Can you work these out from the model? Positions are in its coordinate system, mm. Face numbers are marked on the shaded views. A direction names the side the tool comes from. Round coordinates to 2 decimals unless told otherwise and drop trailing zeros. Loops run counter-clockwise (first coordinate to the right, second up) from the corner with the lowest first, then second, coordinate; pieces in that order, holes last.
from build123d import *

# Parameters (mm, degrees)
SKETCH1_W           = 440
SKETCH1_H           = 327.889328918
BOSS_EXTRUDE1_DEPTH = 120
SKETCH8_W           = 413.828334862
SKETCH8_H           = 293.441910175
CUT_EXTRUDE1_DEPTH  = 110
SKETCH9_R           = 6
SKETCH9_R_2         = 6.017467881
CUT_EXTRUDE4_DEPTH  = 110
SKETCH10_R          = 6
SKETCH10_R_2        = 6.017467881
CUT_EXTRUDE5_DEPTH  = 110


with BuildPart() as part:
    # Sketch1 → Boss-Extrude1 (new body)
    with BuildSketch(Plane(origin=(0, 0, 0), x_dir=(1, 0, 0), z_dir=(0, 1, 0))):
        with Locations((-220, 163.944664459)):
            Rectangle(SKETCH1_W, SKETCH1_H)
    extrude(amount=BOSS_EXTRUDE1_DEPTH)

    # Sketch8 → Cut-Extrude1 (cut)
    with BuildSketch(Plane(origin=(0, 120, 0), x_dir=(1, 0, 0), z_dir=(0, 1, 0))):
        with Locations((-219.994628395, 162.587971533)):
            Rectangle(SKETCH8_W, SKETCH8_H)
    extrude(amount=-CUT_EXTRUDE1_DEPTH, mode=Mode.SUBTRACT)

    # Sketch9 → Cut-Extrude4 (cut)
    with BuildSketch(Plane(origin=(-426.908795826, 0, 0), x_dir=(0, 0, -1), z_dir=(1, 0, 0))):
        with Locations((278, 80)):
            Circle(SKETCH9_R)
        with Locations((278, 26.719560601)):
            Circle(SKETCH9_R)
        with Locations((50, 80)):
            Circle(SKETCH9_R)
        with Locations((50, 26.719560601)):
            Circle(SKETCH9_R_2)
    extrude(amount=-CUT_EXTRUDE4_DEPTH, mode=Mode.SUBTRACT)

    # Sketch10 → Cut-Extrude5 (cut)
    with BuildSketch(Plane(origin=(0, 0, 0), x_dir=(0, 0, -1), z_dir=(1, 0, 0))):
        with Locations((50, 80)):
            Circle(SKETCH10_R)
        with Locations((50, 26.719560601)):
            Circle(SKETCH10_R_2)
        with Locations((278, 26.719560601)):
            Circle(SKETCH10_R)
        with Locations((278, 80)):
            Circle(SKETCH10_R)
    extrude(amount=-CUT_EXTRUDE5_DEPTH, mode=Mode.SUBTRACT)


solid = part.part
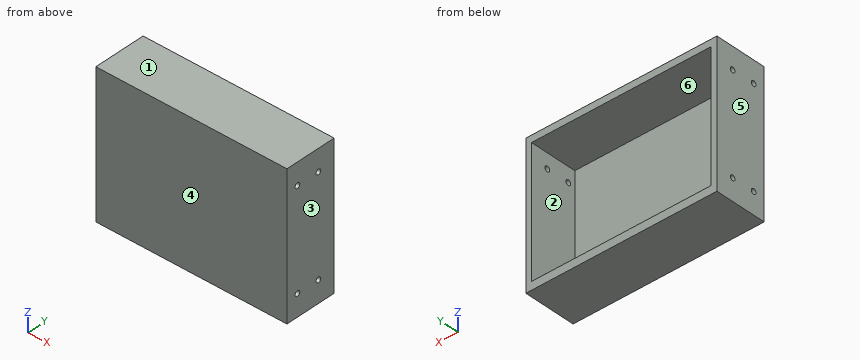
(1) If we mould it in two halves opening along X, with no side actions, what happens to the marked faces 3, 4, 5 and 6? For each: released by +X, released by -X, zero draft, split by the parting line, or undercut.
Worked answers:
face 3: released by +X
face 4: zero draft
face 5: released by -X
face 6: undercut
(2) If we section it at A-A, the plane y = 80: List the corners of the cut face in (x, z) for me, then the cut area to 3 significant figures.
Worked answers:
outline: (-440, -327.89) - (0, -327.89) - (0, -284) - (-13.08, -284) - (-13.08, -309.31) - (-426.91, -309.31) - (-426.91, -284) - (-440, -284) - close; (-440, -272) - (-426.91, -272) - (-426.91, -56) - (-440, -56) - close; (-440, -44) - (-426.91, -44) - (-426.91, -15.87) - (-13.08, -15.87) - (-13.08, -44) - (0, -44) - (0, 0) - (-440, 0) - close; (-13.08, -272) - (0, -272) - (0, -56) - (-13.08, -56) - close
area: 22,200 mm2
(3) If we section it at B-B, the plane z = -50: List the corners of the cut face in (x, y) for me.
Worked answers:
outline: (-440, 0) - (0, 0) - (0, 20.7) - (-13.08, 20.7) - (-13.08, 10) - (-426.91, 10) - (-426.91, 20.7) - (-440, 20.7) - close; (-440, 32.74) - (-426.91, 32.74) - (-426.91, 74) - (-440, 74) - close; (-440, 86) - (-426.91, 86) - (-426.91, 120) - (-440, 120) - close; (-13.08, 32.74) - (0, 32.74) - (0, 74) - (-13.08, 74) - close; (-13.08, 86) - (0, 86) - (0, 120) - (-13.08, 120) - close
(4) If we section it at C-C, the plane x = -131: List the corners of the cut face in (y, z) for me, then the cut area to 3 significant figures.
Worked answers:
outline: (0, -327.89) - (120, -327.89) - (120, -309.31) - (10, -309.31) - (10, -15.87) - (120, -15.87) - (120, 0) - (0, 0) - close
area: 7,070 mm2
(5) For the marked faces 1 and 2, which set-ups out of +Z, -Z, +X, -X, +Y, -Y let a thin tool reach every point of the face, with its end or its side?
Worked answers:
face 1: +Z, +X, -X, +Y, -Y
face 2: +Y
(6) If we section it at D-D, the plane y = 107: List the corners of the cut face in (x, z) for me, then the cut area to 3 significant figures.
Worked answers:
outline: (-440, -327.89) - (0, -327.89) - (0, 0) - (-440, 0) - close; hole (-426.91, -309.31) - (-13.08, -309.31) - (-13.08, -15.87) - (-426.91, -15.87) - close
area: 22,800 mm2
(7) Will this pin go through, and if not, where does the flat tip stop? P1, Ø3, axis at x = -120, z = -220, coming from the +Y side.
Worked answers:
P1: stops at y = 10
(8) If I drill on line 1 (Y direction, x = -9.5, z = -278); line 2 (X direction, y = 41.5, z = -261); line 3 (Z direction, x = -138, y = 69), over which ranges is the centre line in solid material (lowest first)?
Worked answers:
line 1: y = 0 to 20.72, 32.72 to 74, 86 to 120
line 2: x = -440 to -426.91, -13.08 to 0
line 3: z = -327.89 to -309.31, -15.87 to 0
